Autodesk Inventor part; units mm, degrees
ref_plane "YZ Plane" through (0, 0, 0) normal (1, 0, 0) x (0, 1, 0)
ref_plane "XZ Plane" through (0, 0, 0) normal (0, 1, 0) x (-1, 0, 0)
ref_plane "XY Plane" through (0, 0, 0) normal (0, 0, 1) x (1, 0, 0)
sketch "Sketch1" plane through (0, 0, 0) normal (0, 1, 0) x (-1, 0, 0)
  line L0 (0, 0) -> (0, 14.8)
  line L1 (0, 14.8) -> (-2, 14.8)
  line L2 (-2, 14.8) -> (-2, 12.4)
  line L3 (-3, 10.8) -> (-3, 2.8)
  line L4 (-3, 2.8) -> (-5, 2.8)
  line L5 (-5, 2.8) -> (-5, 0)
  line L6 (-5, 0) -> (0, 0)
  line L7 (-1.6, 12) -> (-1.6, 10.8)
  line L8 (-3, 10.8) -> (-1.6, 10.8)
  line L9 (-1.6, 12) -> (-2, 12.4)
  dimension "d0" = 10
  dimension "d1" = 6
  dimension "d2" = 4
  dimension "d4" = 8
  dimension "d5" = 2.8
  dimension "d15" = 4
  dimension "d16" = 3.2
  dimension "d17" = 1.2
  dimension "d18" = 45
revolve "Revolution1" add sketch "Sketch1" angle 360 about axis through (0, 0, 0) along (0, 0, 1)
thread "Thread1"
sketch "Sketch2" plane through (0, 0, 0) normal (0, 0, -1) x (-1, 0, 0)
  line L0 (0, 1.4434) -> (1.25, 0.7217)
  line L1 (1.25, 0.7217) -> (1.25, -0.7217)
  line L2 (1.25, -0.7217) -> (0, -1.4434)
  line L3 (0, -1.4434) -> (-1.25, -0.7217)
  line L4 (-1.25, -0.7217) -> (-1.25, 0.7217)
  line L5 (-1.25, 0.7217) -> (0, 1.4434)
  point P0 (0, 0)
  point P1 (0, 0)
  dimension "d9" = 2.5
extrude "Extrusion1" cut sketch "Sketch2" against normal blind 2
chamfer "Chamfer1" distance 0.43 angle 45 1 edges at (-2, 0, 14.8)
properties part number "DBTSY4-8-4-DHC-PC" material "Stainless Steel AISI 304"
Read the model definition and answer for the solid it produces. Units are mm, in the model's axes. A direction names the side the tool comes from. Give positions to 0.01 mm unless a question says otherwise; leave off trailing zeros. Write each loop counter-clockwise with the first axis right and the second up, starting at its lowest first coordinate (ties: lowest second). Pieces come first, ordered by that corner, then holes. Notation, with made-up numbers: (31, 66) - (59, 66) arc R20 cw to (59, 89) - close; hole circle Ø4 at (42, 58.5). An arc over 180 degrees is marked (long way). Answer in a Markdown table with one row per item. Add a question column.
Item 1: Section B-B, the plane x = -2.25 is taken. Write down the section's boundary in (y, z), and give its area (3 significant figures).
Item 2: Determine the mould class of faces 5 (the face through (0, 2, 13)), 6 (the face through (1.3, -1.3, 10.8)), 7 (the face through (3.3, 0.1, 2.8)) for opening direction Z: pulls with the +Z half, pulls with the -Z half, needs draft (parallel to the pull), parting line crosses it, or undercut.
Item 3: Find the intervals of material crossed by L1, parallel to Z at x = 0.5, y = 1; L2, parallel to Z at x = 3.75, y = 0.25; L3, parallel to Z at x = -1.5, y = 1, in increasing order.
Item 4: A tool of negligible diameter and unlimited length cuts with its end or side. For faces 1 (the face through (-3, 0, 7)), 2 (the face through (-1.27, 0.97, 11.39)), 3 (the face through (1.04, -1.04, 0)), 4 (the face through (0, 0, 2)), from which of +Z, -Z, +X, -X, +Y, -Y can it reach the whole face along a straight path? Write none if from no direction.
Item 5: Section C-C, the plane z = 13.25 is taken. Write down the section's boundary in (x, y).
Item 6: Section D-D, the plane y = -2.5 is taken. Write down the section's boundary in (x, z), and give its area (3 significant figures).
Item 7: Flat-ended cylindrical pins translate along their axes: P1, Ø2, axis at x = -2.5, y = 1, coming from the +Z side; P2, Ø4, axis at x = 0.5, z = 8.5, coming from the +Y side; P3, Ø1, axis at y = -1.5, z = 1.5, coming from the +X side. Find the tip coordinate at first contact, or state that the pin passes through.
Item 8: Section A-A, the plane y = 0 is taken. Write down the section's boundary in (x, z).
Recorded:
| question | item | result |
|---|---|---|
| 1 | outline | (-4.47, 0) - (4.47, 0) - (4.47, 2.8) - (1.98, 2.8) - (1.98, 10.8) - (-1.98, 10.8) - (-1.98, 2.8) - (-4.47, 2.8) - close |
| 1 | area | 56.8 mm2 |
| 2 | face 5 | needs draft |
| 2 | face 6 | undercut |
| 2 | face 7 | pulls with the +Z half |
| 3 | L1 | z = 2 to 14.8 |
| 3 | L2 | z = 0 to 2.8 |
| 3 | L3 | z = 0 to 10.8, 12.2 to 14.57 |
| 4 | face 1 | +Z |
| 4 | face 2 | none |
| 4 | face 3 | -Z, +X, -X, +Y, -Y |
| 4 | face 4 | -Z |
| 5 | outline | circle Ø4 at (0, 0) |
| 6 | outline | (-4.33, 0) - (4.33, 0) - (4.33, 2.8) - (1.66, 2.8) - (1.66, 10.8) - (-1.66, 10.8) - (-1.66, 2.8) - (-4.33, 2.8) - close |
| 6 | area | 50.8 mm2 |
| 7 | P1 | stops at z = 14.68 |
| 7 | P2 | stops at y = 3 |
| 7 | P3 | stops at x = 4.9 |
| 8 | outline | (-5, 0) - (-1.25, 0) - (-1.25, 2) - (1.25, 2) - (1.25, 0) - (5, 0) - (5, 2.8) - (3, 2.8) - (3, 10.8) - (1.6, 10.8) - (1.6, 12) - (2, 12.4) - (2, 14.37) - (1.57, 14.8) - (-1.57, 14.8) - (-2, 14.37) - (-2, 12.4) - (-1.6, 12) - (-1.6, 10.8) - (-3, 10.8) - (-3, 2.8) - (-5, 2.8) - close |
